Model file for the job. Use its own axes, mm. Face numbers are marked on the shaded views. A direction names the side the tool comes from. Round coordinates to 2 decimals unless told otherwise and drop trailing zeros. Loops run counter-clockwise (first coordinate to the right, second up) from the corner with the lowest first, then second, coordinate; pieces in that order, holes last. Notation, with made-up numbers: M 26.25,47.5 L 61.25,47.5 A25 ccw 61.25,78.5 Z; hole C -10,-14.5 d3. An arc over 180 degrees is marked long. Use a Markdown table: item, result. Add a question column.
Q1. Cut at A-A (y = 2.6). Give the cut face in (x, z), plus the area to 3 significant figures.
Q2. Tool access for the marked faces 1 and 2: list every direction of +Z, -Z, +X, -X, +Y, -Y with a clear straight run to the whole face (end or side of a thin tool).
Q3. Probe line 1 (X direction, y = 0.2, z = 0.75); line 2 (X direction, y = 3.75, z = -2); line 3 (Z direction, x = -1, y = 0.7). List the from-to ranges inside material, lowest first. Write a range as from..to.
Q4. Cut at D-D (y = -0.8). Give the cut face in (x, z).
Q5. Mould opens along X. For the marked faces 3, 4, 5 and 6 say: +X half, -X half, draft (parallel to the pull), parting line (faces both ways), or undercut.
Q6. Pin check, flat tips, straight feed: pin 1 (3 mm diameter, centred on x = 0, z = 0, fed in from +Y); pin 2 (2 mm diameter, centred on y = -1.5, z = -2, fed in from +X). Stop position of each tip, or through.
Q7. Cut at C-C (z = -0.5). Give the cut face in (x, y), plus the area to 3 significant figures.
Q8. Cut at B-B (x = 0). Give the cut face in (y, z), plus the area to 3 significant figures.
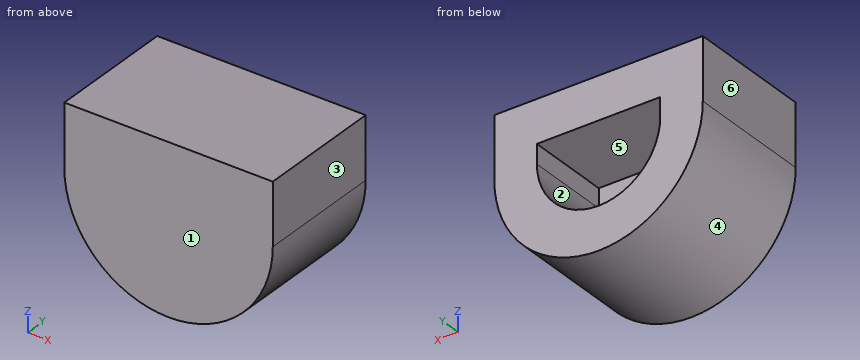
from build123d import *

# Parameters (mm, degrees)
BOSS_EXTRUDE1_DEPTH = 4
BOSS_EXTRUDE2_START = -2
BOSS_EXTRUDE2_DEPTH = 2


with BuildPart() as part:
    # Sketch1 → Boss-Extrude1 (new body)
    with BuildSketch(Plane(origin=(0, 0, 0), x_dir=(1, 0, 0), z_dir=(0, 1, 0))):
        with BuildLine():
            Line((-4.9, 0), (-2.9, 0))
            ThreePointArc((-2.9, 0), (0, 2.9), (2.9, 0))
            Line((2.9, 0), (4.9, 0))
            ThreePointArc((4.9, 0), (0, 4.9), (-4.9, 0))
        make_face()
        with BuildLine():
            Line((4.9, 0), (2.9, 0))
            Line((2.9, 0), (2.9, -0.9))
            Line((2.9, -0.9), (2.75680975, -0.9))
            ThreePointArc((2.75680975, -0.9), (1.702938637, -2.347338919), (0, -2.9))
            Line((0, -2.9), (3.949683532, -2.9))
            ThreePointArc((3.949683532, -2.9), (4.656363887, -1.525868719), (4.9, 0))
        make_face()
        with BuildLine():
            Line((4.9, -2.9), (4.9, 0))
            ThreePointArc((4.9, 0), (4.656363887, -1.525868719), (3.949683532, -2.9))
            Line((3.949683532, -2.9), (4.9, -2.9))
        make_face()
        with BuildLine():
            Line((-2.9, -0.9), (-2.9, 0))
            Line((-2.9, 0), (-4.9, 0))
            ThreePointArc((-4.9, 0), (-4.656363887, -1.525868719), (-3.949683532, -2.9))
            Line((-3.949683532, -2.9), (0, -2.9))
            ThreePointArc((0, -2.9), (-1.702938637, -2.347338919), (-2.75680975, -0.9))
            Line((-2.75680975, -0.9), (-2.9, -0.9))
        make_face()
        with BuildLine():
            ThreePointArc((-3.949683532, -2.9), (-4.656363887, -1.525868719), (-4.9, 0))
            Line((-4.9, 0), (-4.9, -2.9))
            Line((-4.9, -2.9), (-3.949683532, -2.9))
        make_face()
        with BuildLine():
            Line((2.75680975, -0.9), (-2.75680975, -0.9))
            ThreePointArc((-2.75680975, -0.9), (-1.702938637, -2.347338919), (0, -2.9))
            ThreePointArc((0, -2.9), (1.702938637, -2.347338919), (2.75680975, -0.9))
        make_face()
    extrude(amount=BOSS_EXTRUDE1_DEPTH)

    # Sketch1_3 → Boss-Extrude2 (add)
    with BuildSketch(Plane(origin=(0, 0, 0), x_dir=(1, 0, 0), z_dir=(0, 1, 0)).offset(BOSS_EXTRUDE2_START)):
        with BuildLine():
            Line((-4.9, 0), (-2.9, 0))
            ThreePointArc((-2.9, 0), (0, 2.9), (2.9, 0))
            Line((2.9, 0), (4.9, 0))
            ThreePointArc((4.9, 0), (0, 4.9), (-4.9, 0))
        make_face()
        with BuildLine():
            ThreePointArc((-2.75680975, -0.9), (-2.863978725, -0.455659809), (-2.9, 0))
            Line((-2.9, 0), (-2.9, -0.9))
            Line((-2.9, -0.9), (-2.75680975, -0.9))
        make_face()
        with BuildLine():
            Line((2.9, -0.9), (2.9, 0))
            ThreePointArc((2.9, 0), (2.863978725, -0.455659809), (2.75680975, -0.9))
            Line((2.75680975, -0.9), (2.9, -0.9))
        make_face()
        with BuildLine():
            ThreePointArc((2.9, 0), (0, 2.9), (-2.9, 0))
            Line((-2.9, 0), (2.9, 0))
        make_face()
        with BuildLine():
            Line((2.9, 0), (-2.9, 0))
            ThreePointArc((-2.9, 0), (-2.863978725, -0.455659809), (-2.75680975, -0.9))
            Line((-2.75680975, -0.9), (2.75680975, -0.9))
            ThreePointArc((2.75680975, -0.9), (2.863978725, -0.455659809), (2.9, 0))
        make_face()
        with BuildLine():
            Line((-2.9, -0.9), (-2.9, 0))
            Line((-2.9, 0), (-4.9, 0))
            ThreePointArc((-4.9, 0), (-4.656363887, -1.525868719), (-3.949683532, -2.9))
            Line((-3.949683532, -2.9), (0, -2.9))
            ThreePointArc((0, -2.9), (-1.702938637, -2.347338919), (-2.75680975, -0.9))
            Line((-2.75680975, -0.9), (-2.9, -0.9))
        make_face()
        with BuildLine():
            Line((4.9, 0), (2.9, 0))
            Line((2.9, 0), (2.9, -0.9))
            Line((2.9, -0.9), (2.75680975, -0.9))
            ThreePointArc((2.75680975, -0.9), (1.702938637, -2.347338919), (0, -2.9))
            Line((0, -2.9), (3.949683532, -2.9))
            ThreePointArc((3.949683532, -2.9), (4.656363887, -1.525868719), (4.9, 0))
        make_face()
        with BuildLine():
            Line((4.9, -2.9), (4.9, 0))
            ThreePointArc((4.9, 0), (4.656363887, -1.525868719), (3.949683532, -2.9))
            Line((3.949683532, -2.9), (4.9, -2.9))
        make_face()
        with BuildLine():
            ThreePointArc((-3.949683532, -2.9), (-4.656363887, -1.525868719), (-4.9, 0))
            Line((-4.9, 0), (-4.9, -2.9))
            Line((-4.9, -2.9), (-3.949683532, -2.9))
        make_face()
        with BuildLine():
            Line((2.75680975, -0.9), (-2.75680975, -0.9))
            ThreePointArc((-2.75680975, -0.9), (-1.702938637, -2.347338919), (0, -2.9))
            ThreePointArc((0, -2.9), (1.702938637, -2.347338919), (2.75680975, -0.9))
        make_face()
    extrude(amount=BOSS_EXTRUDE2_DEPTH)


solid = part.part
Checked values:
| question | item | result |
|---|---|---|
| 1 | outline | M -4.9,0 A4.9 ccw 4.9,0 L 4.9,2.9 L -4.9,2.9 Z; hole M -2.9,0 A2.9 ccw 2.9,0 L 2.9,0.9 L -2.9,0.9 Z |
| 1 | area | 47.7 mm^2 |
| 2 | face 1 | +Z, -Z, +X, -X, -Y |
| 2 | face 2 | +Y |
| 3 | line 1 | x = -4.9..-2.9, 2.9..4.9 |
| 3 | line 2 | x = -4.47..-2.1, 2.1..4.47 |
| 3 | line 3 | z = -4.8..-2.72, 0.9..2.9 |
| 4 | outline | M -4.9,0 A4.9 ccw 4.9,0 L 4.9,2.9 L -4.9,2.9 Z |
| 5 | face 3 | +X half |
| 5 | face 4 | parting line |
| 5 | face 5 | undercut |
| 5 | face 6 | -X half |
| 6 | pin 1 | stops at y = 4 |
| 6 | pin 2 | stops at x = 4.8 |
| 7 | outline | M -4.87,-2 L 4.87,-2 L 4.87,4 L 2.86,4 L 2.86,0 L -2.86,0 L -2.86,4 L -4.87,4 Z |
| 7 | area | 35.6 mm^2 |
| 8 | outline | M -2,-4.9 L 4,-4.9 L 4,-2.9 L 0,-2.9 L 0,0.9 L 4,0.9 L 4,2.9 L -2,2.9 Z |
| 8 | area | 31.6 mm^2 |
